```python
from build123d import *

# Parameters (mm, degrees)
SKETCH3_W           = 32.5
SKETCH3_H           = 6
CHAMFER2_SIZE       = 2
SKETCH4_R           = 2.5
BOSS_EXTRUDE1_DEPTH = 13.8
CIRPATTERN1_COUNT   = 6
CHAMFER3_SIZE       = 2
CHAMFER4_SIZE       = 0.25


with BuildPart() as part:
    # Sketch3 → Revolve1 (revolve)
    with BuildSketch(Plane(origin=(0, 0, 0), x_dir=(0, 0, -1), z_dir=(1, 0, 0))):
        with Locations((-16.25, 28)):
            Rectangle(SKETCH3_W, SKETCH3_H)
    revolve(axis=Axis((0, 0, 0), (0, -1, 0)))

    # Chamfer2
    chamfer2_edges = [part.edges().sort_by_distance(p)[0] for p in [
        (0, 31, -32.5),
    ]]
    chamfer(chamfer2_edges, length=CHAMFER2_SIZE)

    # Sketch4 → Boss-Extrude1 (add)
    with BuildSketch(Plane.XZ.offset(-25)):
        with Locations(Location((0, 26.5, 0), (0, 0, 180))):
            Circle(SKETCH4_R)
    boss_extrude1 = extrude(amount=BOSS_EXTRUDE1_DEPTH)

    # CirPattern1: Boss-Extrude1 ×6 about axis
    cirpattern1_axis = Axis((0, 0, 0), (0, 1, 0))
    for i in range(1, CIRPATTERN1_COUNT):
        add(boss_extrude1.rotate(cirpattern1_axis, i * 360 / CIRPATTERN1_COUNT))

    # Chamfer3
    chamfer3_edges = [part.edges().sort_by_distance(p)[0] for p in [
        (2.5, 25, 26.5),
        (24.1996732, 25, 11.084936491),
        (21.6996732, 25, -15.415063509),
        (-2.5, 25, -26.5),
        (-24.1996732, 25, -11.084936491),
        (-21.6996732, 25, 15.415063509),
    ]]
    chamfer(chamfer3_edges, length=CHAMFER3_SIZE)

    # Chamfer4
    chamfer4_edges = [part.edges().sort_by_distance(p)[0] for p in [
        (0, 25, -32.5),
    ]]
    chamfer(chamfer4_edges, length=CHAMFER4_SIZE)


solid = part.part
```
Can you work these out from the model? Positions are in its coordinate system, mm. A direction names the side the tool comes from. Round coordinates to 2 decimals unless told otherwise and drop trailing zeros. Order: outer loops, then holes, each group sorted by start corner. A loop starts at its lowest first (then second) coordinate and runs counter-clockwise, first axis right, second up. Notation, with made-up numbers: (60, 50.25) -> (73, 50.25) arc R14 ccw to (73, 54.25) -> close; hole circle Ø5 at (34.5, 49.25). An arc over 180 degrees is marked (long way). Return JSON: item names as keys, results as strings. Group by question number.
1. Which directions (+Z, -Z, +X, -X, +Y, -Y) give clear straight access to the entire face, cutting with the end or side of a thin tool? Please do faces 4 (the face through (23.28, 17.18, -15.73)), 5 (the face through (-23, 11.2, -13)).
2. I need wall thicknesses on line 1 (Y direction, x = -5, z = -29); line 2 (Z direction, x = 1, y = 13); line 3 (X direction, y = 18.75, z = 15). Which ranges of each line are inside material? Lowest first, please. Write a range as [from, to].
3. If we section it at A-A, the plane y = 19.5: Write out the boundary of the cut face in (x, z).
4. Will these pins go through, and if not, where does the flat tip stop? pin 1 (4 mm diameter, centred on x = 16.5, y = 27.5, fed in from +Z); pin 2 (1 mm diameter, centred on y = 23.5, z = 14, fed in from -X); pin 3 (1 mm diameter, centred on x = 10, y = 27, fed in from -Z).
5. We'd pull the mould along Z, two halves only. Please class faces 1 (the face through (-9.76, 27.15, 31)), 2 (the face through (0, 11.2, 26)), 3 (the face through (-24.1, 17.18, -11.03)): released by +Z, released by -Z, zero draft, split by the parting line, or undercut.
Output values:
{
 "1": {"face 4": "-Y", "face 5": "+Z, -Z, +X, -X, -Y"},
 "2": {"line 1": "[25, 31]", "line 2": "[-28.79, -24.21], [24.21, 28.79]", "line 3": "[-24.74, -21.16], [21.16, 24.74]"},
 "3": {"outline": "circle Ø5 at (-22.95, -13.25); circle Ø5 at (-22.95, 13.25); circle Ø5 at (0, -26.5); circle Ø5 at (0, 26.5); circle Ø5 at (22.95, -13.25); circle Ø5 at (22.95, 13.25)"},
 "4": {"pin 1": "z = 29.09", "pin 2": "x = -26.38", "pin 3": "z = -31.08"},
 "5": {"face 1": "split by the parting line", "face 2": "zero draft", "face 3": "undercut"}
}
